```python
from build123d import *

# Parameters (mm, degrees)
SKETCH003_W             = 95
SKETCH003_H             = 27
PAD002_DEPTH            = 2
SKETCH004_R             = 1.3
POCKET001_DEPTH         = 2
FILLET002_R             = 3
SKETCH005_W             = 9.2
SKETCH005_H             = 11.4
POCKET002_DEPTH         = 2
BODY001_PLACEMENT_ANGLE = 180


with BuildPart() as part:
    # Sketch003 → Pad002 (new body)
    with BuildSketch(Plane.XY):
        Rectangle(SKETCH003_W, SKETCH003_H)
    extrude(amount=PAD002_DEPTH)

    # Sketch004 (on Face6 of Pad002) → Pocket001 (cut)
    with BuildSketch(Plane.XY.offset(2)):
        with Locations((-44.5, 10.5)):
            Circle(SKETCH004_R)
        with Locations((44.5, 10.5)):
            Circle(SKETCH004_R)
        with Locations((44.5, -10.5)):
            Circle(SKETCH004_R)
        with Locations((-44.5, -10.5)):
            Circle(SKETCH004_R)
    extrude(amount=-POCKET001_DEPTH, mode=Mode.SUBTRACT)

    # Fillet002
    fillet002_edges = [part.edges().sort_by_distance(p)[0] for p in [
        (-47.5, -13.5, 1),
        (47.5, -13.5, 1),
        (47.5, 13.5, 1),
        (-47.5, 13.5, 1),
    ]]
    fillet(fillet002_edges, radius=FILLET002_R)

    # Sketch005 (on Face5 of Fillet002) → Pocket002 (cut)
    with BuildSketch(Plane.XY.offset(2)):
        with Locations((31.3, 1.1)):
            Rectangle(SKETCH005_W, SKETCH005_H)
    extrude(amount=-POCKET002_DEPTH, mode=Mode.SUBTRACT)


with BuildPart() as part_1:
    # Body001 placement: moved
    add(part.part.moved(Location((0, -1, -0.4))).rotate(Axis((0, -1, -0.4), (0, 1, 0)), BODY001_PLACEMENT_ANGLE))


solid = part_1.part
```
Source: CAD feature listing. Evaluate the final solid. Frame: model axes, mm. A direction names the side the tool comes from. Coordinates: 2 decimals unless noted, no trailing zeros. Loops run counter-clockwise (first coordinate to the right, second up) from the corner with the lowest first, then second, coordinate; pieces in that order, holes last. Notation, with made-up numbers: M 69,65 L 85,65 A27 cw 85,81 Z; hole C -1.75,57.25 d3. An arc over 180 degrees is marked long. Use a Markdown table: item, result. Add a question column.
Q1. Access query for faces 4 (the flat face through (-31, 5.8, -1)), 5 (the cylindrical face through (-46.6, -13.64, -1.41)). Directions: +Z, -Z, +X, -X, +Y, -Y. A direction counts if a zero-diameter tool reaches every point of the face in a straight line with its end or side. Return the directions, or none.
Q2. Draft query along Y for faces 1 (the flat face through (1, -14.5, -1)), 2 (the flat face through (-26.7, 0, -1)), 3 (the flat face through (1, -1, -0.4)). Return one class per face: pulls with the +Y half, pulls with the -Y half, needs draft (parallel to the pull), parting line crosses it, or undercut.
Q3. Section query A-A, the plane y = -1.75. Return loops of the section in (x, z), and give its area (3 significant figures).
Q4. Section query B-B, the plane z = -1.3. Return loops of the section in (x, y).
Q5. Material intervals for L1, parallel to Y at x = 44.5, z = -1.8; L2, parallel to X at y = 2.75, z = -1.9; L3, parallel to Y at x = -33, z = -0.7, sorted ascending.
Q6. First-contact query: pin 1 (1.6 mm diameter, centred on x = 44.5, y = 9.5, fed in from +Z). Flat tip, straight axial feed; report the tip coordinate or a pass-through.
Result:
| question | item | result |
|---|---|---|
| 1 | face 4 | +Z, -Z |
| 1 | face 5 | +Z, -Z, -X, -Y |
| 2 | face 1 | pulls with the -Y half |
| 2 | face 2 | undercut |
| 2 | face 3 | needs draft |
| 3 | outline | M -47.5,-2.4 L -35.9,-2.4 L -35.9,-0.4 L -47.5,-0.4 Z; M -26.7,-2.4 L 47.5,-2.4 L 47.5,-0.4 L -26.7,-0.4 Z |
| 3 | area | 172 mm2 |
| 4 | outline | M -47.5,-11.5 A3 ccw -44.5,-14.5 L 44.5,-14.5 A3 ccw 47.5,-11.5 L 47.5,9.5 A3 ccw 44.5,12.5 L -44.5,12.5 A3 ccw -47.5,9.5 Z; hole C -44.5,-11.5 d2.6; hole C -44.5,9.5 d2.6; hole M -35.9,-5.6 L -26.7,-5.6 L -26.7,5.8 L -35.9,5.8 Z; hole C 44.5,-11.5 d2.6; hole C 44.5,9.5 d2.6 |
| 5 | L1 | y = -14.5 to -12.8, -10.2 to 8.2, 10.8 to 12.5 |
| 5 | L2 | x = -47.5 to -35.9, -26.7 to 47.5 |
| 5 | L3 | y = -14.5 to -5.6, 5.8 to 12.5 |
| 6 | pin 1 | passes through |
